```python
from build123d import *

# Parameters (mm, degrees)
F0_W     = 79.736687
F0_H     = 79.736683
F1_DEPTH = 7.112
F3_DEPTH = 6.35
F4_SIZE  = 5.08
F6_D     = 25.4
F8_D     = 20.32
F5_R     = 12.951628
F9_DEPTH = 4.572


with BuildPart() as f1:
    # F0 (on Top) → F1 (new body)
    with BuildSketch(Plane.XY):
        with Locations((0.753854, 7.008081)):
            Rectangle(F0_W, F0_H)
    extrude(amount=F1_DEPTH)

    # F2 (on face) → F3 (cut)
    with BuildSketch(Plane.XY.offset(7.112)):
        with BuildLine():
            ThreePointArc((12.293341, -29.39476), (31.214057, -15.396734), (38.42256, 7.008081))
            ThreePointArc((38.42256, 7.008081), (38.359097, 9.215515), (38.168919, 11.415657))
            ThreePointArc((38.168919, 11.415657), (23.100575, 18.141586), (27.227051, 34.118611))
            ThreePointArc((27.227051, 34.118611), (0.347081, 45.429074), (-26.732835, 34.606064))
            ThreePointArc((-26.732835, 34.606064), (-22.915627, 30.093116), (-21.544947, 24.343419))
            ThreePointArc((-21.544947, 24.343419), (-26.733198, 14.080507), (-38.073768, 12.173477))
            ThreePointArc((-38.073768, 12.173477), (-32.65258, -13.242897), (-12.293341, -29.39476))
            ThreePointArc((-12.293341, -29.39476), (0, -20.087793), (12.293341, -29.39476))
        make_face()
    extrude(amount=-F3_DEPTH, mode=Mode.SUBTRACT)

    # F4
    f4_edges = [f1.edges().sort_by_distance(p)[0] for p in [
        (40.622197, 46.876423, 3.556),
        (-39.11449, 46.876423, 3.556),
        (40.622197, -32.86026, 3.556),
        (-39.11449, -32.86026, 3.556),
    ]]
    chamfer(f4_edges, length=F4_SIZE)

    # F6 (through all)
    with Locations(Plane.XY.offset(7.112)):
        with Locations((0, 7.008081)):
            Hole(F6_D / 2)

    # F8 (through all)
    with Locations(Plane.XY.offset(7.112)):
        with Locations((0, 46.382606)):
            Hole(F8_D / 2)

    # F5 (on face) + F0 (on Top) → F9 (cut)
    with BuildSketch(Plane.XY.offset(7.112)):
        with BuildLine():
            ThreePointArc((-12.293341, -29.39476), (0, -20.087793), (12.293341, -29.39476))
            ThreePointArc((12.293341, -29.39476), (31.214057, -15.396734), (38.42256, 7.008081))
            ThreePointArc((38.42256, 7.008081), (38.359097, 9.215515), (38.168919, 11.415657))
            ThreePointArc((38.168919, 11.415657), (23.100575, 18.141586), (27.227051, 34.118611))
            ThreePointArc((27.227051, 34.118611), (0.347081, 45.429074), (-26.732835, 34.606064))
            ThreePointArc((-26.732835, 34.606064), (-22.915627, 30.093116), (-21.544947, 24.343419))
            ThreePointArc((-21.544947, 24.343419), (-26.733198, 14.080507), (-38.073768, 12.173477))
            ThreePointArc((-38.073768, 12.173477), (-32.65258, -13.242897), (-12.293341, -29.39476))
        make_face()
        with Locations((0, 7.62)):
            Circle(F5_R, mode=Mode.SUBTRACT)
    with BuildSketch(Plane.XY):
        with Locations((0.753854, 7.008081)):
            Rectangle(F0_W, F0_H)
    extrude(amount=-F9_DEPTH, mode=Mode.SUBTRACT)


solid = f1.part
```
Geometry check sheet. Reference: the model listing, model coordinates, mm. Give positions to 0.01 mm unless a question says otherwise; leave off trailing zeros. Loops run counter-clockwise (first coordinate to the right, second up) from the corner with the lowest first, then second, coordinate; pieces in that order, holes last. Notation, with made-up numbers: M 69.25,15.5 L 123.25,15.5 A9 ccw 123.25,24.5 Z; hole C -2,66.25 d8. An arc over 180 degrees is marked long. Write item = value, one per line.
(1) Gauge pin test, flat ends, axial feed: pin 1 Ø4 at (x, y) = (7, 1) entering from -Z; pin 2 Ø22 at (x, y) = (15.5, -9) entering from +Z. Record the tip position at first contact, or that the pin passes through.
Answer below:
pin_1 = through
pin_2 = 0.76
(2) Release check for a two-part mould opening along Y. For faces 1 (the face through (-26, 16, 7.112)), 2 (the face through (38.12, 44.3, 3.51)), 3 (the face through (31.018, -15.668, 3.981)) record: released by +Y, released by -Y, zero draft, split by the parting line, or undercut.
Answer below:
face_1 = zero draft
face_2 = released by +Y
face_3 = undercut
(3) Sectioned sample at D-D, the plane x = -20. Record the cut outline in (y, z).
Answer below:
outline = M -32.86,0 L 46.88,0 L 46.88,7.11 L 39.81,7.11 L 39.81,0.76 L -25.8,0.76 L -25.8,7.11 L -32.86,7.11 Z
(4) Sectioned sample at C-C, the plane x = 0. Record the cut outline in (y, z), plus the area to 3 significant figures.
Answer below:
outline = M -32.86,0 L -5.69,0 L -5.69,0.76 L -20.09,0.76 L -20.09,7.11 L -32.86,7.11 Z; M 19.71,0 L 36.22,0 L 36.22,0.76 L 19.71,0.76 Z
area = 114 mm2
(5) Sectioned sample at A-A, the plane z = 2.5. Record the cut outline in (x, y).
Answer below:
outline = M -39.11,-27.78 L -34.03,-32.86 L 35.54,-32.86 L 40.62,-27.78 L 40.62,41.8 L 35.54,46.88 L 10.15,46.88 A10.16 cw 9.91,44.13 A38.42 cw 27.23,34.12 A12.78 ccw 38.17,11.42 A38.42 cw 38.42,7.01 A38.42 cw 12.29,-29.39 A12.77 ccw -12.29,-29.39 A38.42 cw -38.07,12.17 A12.74 ccw -21.54,24.34 A12.74 ccw -26.73,34.61 A38.42 cw -9.91,44.13 A10.16 cw -10.15,46.88 L -34.03,46.88 L -39.11,41.8 Z
(6) Material ranges on line 1 (Y direction, x = 0, z = 0.55); line 2 (X direction, y = 8, z = 2.25); line 3 (X direction, y = -27, z = 5.5), recorded low to high. Write a range as [from, to].
Answer below:
line_1 = [-32.86, -5.69], [19.71, 36.22]
line_2 = [-39.11, -38.41], [38.41, 40.62]
line_3 = [-39.11, -17.88], [-11.35, 11.35], [17.88, 40.62]
(7) Sectioned sample at B-B, the plane y = 3. Record the cut outline in (x, z), plus the area to 3 significant figures.
Answer below:
outline = M -39.11,0 L -12.05,0 L -12.05,0.76 L -38.21,0.76 L -38.21,7.11 L -39.11,7.11 Z; M 12.05,0 L 40.62,0 L 40.62,7.11 L 38.21,7.11 L 38.21,0.76 L 12.05,0.76 Z
area = 63.4 mm2
